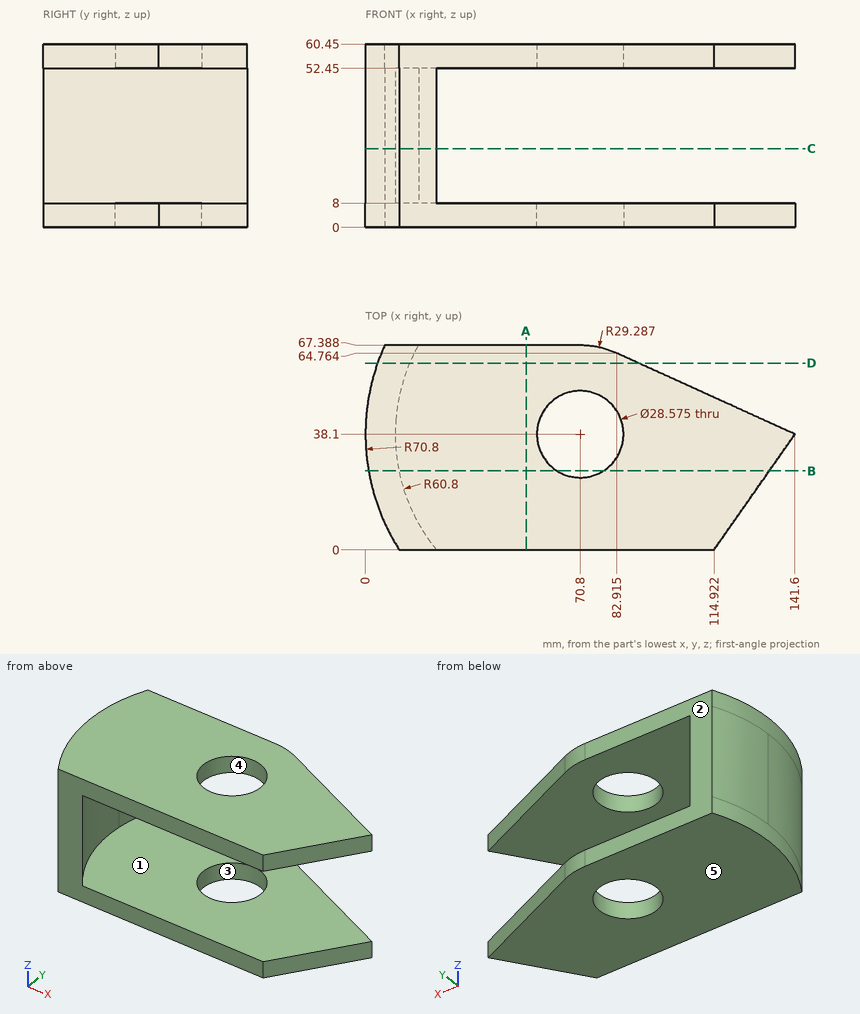
Geometry check sheet. Reference: drawing and pictorial views, mm from the part's lowest x, y, z. A direction names the side the tool comes from. Round coordinates to 2 decimals unless told otherwise and drop trailing zeros. Loops run counter-clockwise (first coordinate to the right, second up) from the corner with the lowest first, then second, coordinate; pieces in that order, holes last. Notation, with made-up numbers: M 43.25,38 L 60.25,38 A31 ccw 60.25,66 Z; hole C 84.25,14 d7. An arc over 180 degrees is marked long. One line per item, written item: value.
(1) Sectioned sample at B-B, the plane y = 26. Record the cut outline in (x, z).
Computed values:
outline: M 1.04,0 L 63.2,0 L 63.2,8 L 11.22,8 L 11.22,52.45 L 63.2,52.45 L 63.2,60.45 L 1.04,60.45 Z; M 78.4,0 L 133.13,0 L 133.13,8 L 78.4,8 Z; M 78.4,52.45 L 133.13,52.45 L 133.13,60.45 L 78.4,60.45 Z
(2) Sectioned sample at C-C, the plane z = 26. Record the cut outline in (x, y) (1 decimal), then the cut area to 3 significant figures.
Computed values:
outline: M 6.3,67.4 A70.8 ccw 11.1,0 L 23.4,0 A60.8 cw 17.5,67.4 Z
area: 710 mm^2
(3) Sectioned sample at D-D, the plane y = 61.5. Record the cut outline in (x, z), then the cut area to 3 significant figures.
Computed values:
outline: M 3.98,0 L 90.1,0 L 90.1,8 L 14.68,8 L 14.68,52.45 L 90.1,52.45 L 90.1,60.45 L 3.98,60.45 Z
area: 1,850 mm^2
(4) Access from +Z, -Z, +X, -X, +Y, -Y to the whole of each face (thin tool, end or side, straight path). Record for the marked faces 1 and 2.
Computed values:
face 1: +X
face 2: +Z, -Z, +X, -X, +Y
(5) Release check for a two-part mould opening along X. For the marked faces 3, 4 and 5 record: +X half, -X half, draft (parallel to the pull), parting line (faces both ways), or undercut.
Computed values:
face 3: undercut
face 4: undercut
face 5: draft
(6) Sectioned sample at A-A, the plane x = 53. Record the cut outline in (y, z), then the cut area to 3 significant figures.
Computed values:
outline: M 0,0 L 67.39,0 L 67.39,8 L 0,8 Z; M 0,52.45 L 67.39,52.45 L 67.39,60.45 L 0,60.45 Z
area: 1,080 mm^2
(7) Depth check by flat-ended pin: pin 1 Ø6 at (y, z) = (49.5, 27.5) entering from +X; pin 2 Ø6 at (y, z) = (57, 46.5) entering from -X; pin 3 Ø6 at (y, z) = (8.5, 48.5) entering from +X. Enter the tip coordinate at first touch or a pass-through.
Computed values:
pin 1: stops at x = 11.73
pin 2: stops at x = 1.81
pin 3: stops at x = 19.48
(8) Thickness scan on line 1 (Z direction, x = 88, y = 13.5); line 2 (Y direction, x = 70, z = 55) (1 decimal); line 3 (X direction, y = 15.5, z = 55) (1 decimal). Record the ranges inside material, lowest first.
Computed values:
line 1: z = 0 to 8, 52.45 to 60.45
line 2: y = 0 to 23.8, 52.4 to 67.4
line 3: x = 3.7 to 125.8
